from build123d import *

# Parameters (mm, degrees)
SALIENTE_EXTRUIR1_DEPTH = 6.35
CROQUIS2_R              = 37.5
CROQUIS2_R_2            = 3
CORTAR_EXTRUIR1_DEPTH   = 6.35


with BuildPart() as part:
    # Croquis1 → Saliente-Extruir1 (new body)
    with BuildSketch(Plane.XY):
        Polygon((-50.356515977, -4.516705607), (-50.356515977, -125.866705607), (100.993484023, -125.866705607), (100.993484023, 25.483294393), (-20.356515977, 25.483294393), (-20.356515977, -4.516705607), align=None)
    extrude(amount=SALIENTE_EXTRUIR1_DEPTH)

    # Croquis2 → Cortar-Extruir1 (cut)
    with BuildSketch(Plane.XY.offset(6.35)):
        with Locations((28.493484023, -53.366705607)):
            Circle(CROQUIS2_R)
        with Locations((-8.006515977, -18.366705607)):
            Circle(CROQUIS2_R_2)
        with Locations((-8.006515977, -88.366705607)):
            Circle(CROQUIS2_R_2)
        with Locations(Location((64.993484023, -18.366705607, 0), (0, 0, 180))):
            Circle(CROQUIS2_R_2)
        with Locations(Location((64.993484023, -88.366705607, 0), (0, 0, 180))):
            Circle(CROQUIS2_R_2)
    extrude(amount=-CORTAR_EXTRUIR1_DEPTH, mode=Mode.SUBTRACT)


solid = part.part
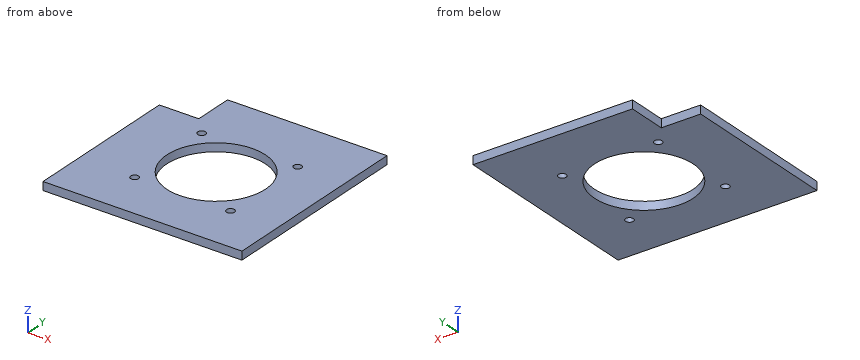
Verification items for the finished model (mm, model axes). Give positions to 0.01 mm unless a question says otherwise; leave off trailing zeros. Write each loop counter-clockwise with the first axis right and the second up, starting at its lowest first coordinate (ties: lowest second). Pieces come first, ordered by that corner, then holes. Notation, with made-up numbers: M 10.5,1 L 37.5,1 A21 cw 37.5,9 Z; hole C 21.25,61 d4. An arc over 180 degrees is marked long. Put each result on its own line as item: value. Start each with the question number.
1. Section check B-B (x = 37). Record the cut outline in (y, z), and give its area (3 significant figures).
2. Go/stop test with a flat-tipped pin: pin 1 Ø1.9 at (x, z) = (-31.5, 2.5) entering from +Y. Record where the tip stops, or that it passes through.
3. Section check C-C (z = 4.25). Record the cut outline in (x, y), and give its area (3 significant figures).
4. Scan lines: line 1 along X through (y, z) = (-4, 5.5); line 2 along Y through (x, z) = (-25.5, 4.5); line 3 along X through (y, z) = (-69, 4). Record each from-to range of solid material in increasing order. Write a range as [from, to].
5. Section check D-D (x = -32). Record the cut outline in (y, z).
6. Section check A-A (y = -71). Record the cut outline in (x, z), and give its area (3 significant figures).
Answer list:
1. outline: M -125.87,0 L -89.89,0 L -89.89,6.35 L -125.87,6.35 Z; M -16.84,0 L 25.48,0 L 25.48,6.35 L -16.84,6.35 Z
1. area: 497 mm2
2. pin 1: y = -4.52
3. outline: M -50.36,-125.87 L 100.99,-125.87 L 100.99,25.48 L -20.36,25.48 L -20.36,-4.52 L -50.36,-4.52 Z; hole C -8.01,-88.37 d6; hole C -8.01,-18.37 d6; hole C 28.49,-53.37 d75; hole C 64.99,-88.37 d6; hole C 64.99,-18.37 d6
3. area: 17,500 mm2
4. line 1: [-20.36, 100.99]
4. line 2: [-125.87, -4.52]
4. line 3: [-50.36, -5.59], [62.58, 100.99]
5. outline: M -125.87,0 L -4.52,0 L -4.52,6.35 L -125.87,6.35 Z
6. outline: M -50.36,0 L -4.6,0 L -4.6,6.35 L -50.36,6.35 Z; M 61.59,0 L 100.99,0 L 100.99,6.35 L 61.59,6.35 Z
6. area: 541 mm2
